Here's how the part is built. I have some questions about the finished solid (model axes, mm). Face numbers are marked on the shaded views. A direction names the side the tool comes from. Coordinates: 2 decimals unless noted, no trailing zeros. Write each loop counter-clockwise with the first axis right and the second up, starting at its lowest first coordinate (ties: lowest second). Pieces come first, ordered by that corner, then holes. Notation, with made-up numbers: M 25.25,88 L 34.25,88 A29 cw 34.25,109 Z; hole C 59.5,47.5 d4. An arc over 180 degrees is marked long. Use a Markdown table: item, result.
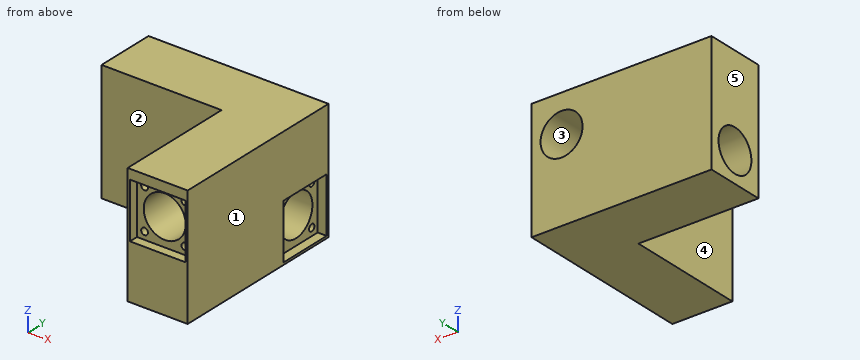
```python
from build123d import *

# Parameters (mm, degrees)
F0_W      = 120
F0_H      = 120
F1_DEPTH  = 80
F2_W      = 37
F2_H      = 37
F2_R      = 2.25
F2_R_2    = 14
F3_DEPTH  = 6
F4_DEPTH  = 120.001
F5_DEPTH  = 25
F6_W      = 37
F6_H      = 37
F6_R      = 2.25
F6_R_2    = 14
F7_DEPTH  = 6
F8_DEPTH  = 120.001
F9_DEPTH  = 25
F10_W     = 80
F10_H     = 80
F11_DEPTH = 80.001


with BuildPart() as f1:
    # F0 (on Top) → F1 (new body)
    with BuildSketch(Plane.XY):
        Rectangle(F0_W, F0_H)
    extrude(amount=F1_DEPTH)

    # F2 (on face) → F3 (cut)
    with BuildSketch(Plane.XZ.offset(60)):
        with Locations((40, 55)):
            Rectangle(F2_W, F2_H)
        with Locations((26.564971, 41.564971)):
            Circle(F2_R, mode=Mode.SUBTRACT)
        with Locations((53.435029, 41.564971)):
            Circle(F2_R, mode=Mode.SUBTRACT)
        with Locations((26.564971, 68.435029)):
            Circle(F2_R, mode=Mode.SUBTRACT)
        with Locations((40, 55)):
            Circle(F2_R_2, mode=Mode.SUBTRACT)
        with Locations((53.435029, 68.435029)):
            Circle(F2_R, mode=Mode.SUBTRACT)
        with Locations((26.564971, 68.435029)):
            Circle(F2_R)
        with Locations((40, 55)):
            Circle(F2_R_2)
        with Locations((53.435029, 68.435029)):
            Circle(F2_R)
        with Locations((53.435029, 41.564971)):
            Circle(F2_R)
        with Locations((26.564971, 41.564971)):
            Circle(F2_R)
    extrude(amount=-F3_DEPTH, mode=Mode.SUBTRACT)

    # F2 (on face) → F4 (cut, through all)
    with BuildSketch(Plane.XZ.offset(60)):
        with Locations((40, 55)):
            Circle(F2_R_2)
    extrude(amount=-F4_DEPTH, mode=Mode.SUBTRACT)

    # F2 (on face) → F5 (cut)
    with BuildSketch(Plane.XZ.offset(60)):
        with Locations((26.564971, 68.435029)):
            Circle(F2_R)
        with Locations((53.435029, 68.435029)):
            Circle(F2_R)
        with Locations((53.435029, 41.564971)):
            Circle(F2_R)
        with Locations((26.564971, 41.564971)):
            Circle(F2_R)
    extrude(amount=-F5_DEPTH, mode=Mode.SUBTRACT)

    # F6 (on face) → F7 (cut)
    with BuildSketch(Plane.YZ.offset(60)):
        with Locations((40, 20)):
            Rectangle(F6_W, F6_H)
        with Locations((26.564971, 6.564971)):
            Circle(F6_R, mode=Mode.SUBTRACT)
        with Locations((53.435029, 6.564971)):
            Circle(F6_R, mode=Mode.SUBTRACT)
        with Locations((26.564971, 33.435029)):
            Circle(F6_R, mode=Mode.SUBTRACT)
        with Locations((40, 20)):
            Circle(F6_R_2, mode=Mode.SUBTRACT)
        with Locations((53.435029, 33.435029)):
            Circle(F6_R, mode=Mode.SUBTRACT)
        with Locations((40, 20)):
            Circle(F6_R_2)
        with Locations((26.564971, 33.435029)):
            Circle(F6_R)
        with Locations((53.435029, 33.435029)):
            Circle(F6_R)
        with Locations((53.435029, 6.564971)):
            Circle(F6_R)
        with Locations((26.564971, 6.564971)):
            Circle(F6_R)
    extrude(amount=-F7_DEPTH, mode=Mode.SUBTRACT)

    # F6 (on face) → F8 (cut, through all)
    with BuildSketch(Plane.YZ.offset(60)):
        with Locations((40, 20)):
            Circle(F6_R_2)
    extrude(amount=-F8_DEPTH, mode=Mode.SUBTRACT)

    # F6 (on face) → F9 (cut)
    with BuildSketch(Plane.YZ.offset(60)):
        with Locations((26.564971, 33.435029)):
            Circle(F6_R)
        with Locations((53.435029, 33.435029)):
            Circle(F6_R)
        with Locations((53.435029, 6.564971)):
            Circle(F6_R)
        with Locations((26.564971, 6.564971)):
            Circle(F6_R)
    extrude(amount=-F9_DEPTH, mode=Mode.SUBTRACT)

    # F10 (on face) → F11 (cut, through all)
    with BuildSketch(Plane.XY.offset(80)):
        with Locations((-20, -20)):
            Rectangle(F10_W, F10_H)
    extrude(amount=-F11_DEPTH, mode=Mode.SUBTRACT)


solid = f1.part
```
1. We'd pull the mould along X, two halves only. Please class the marked faces 1, 2 and 3: +X half, -X half, draft (parallel to the pull), parting line (faces both ways), or undercut.
Answers follow:
| item | result |
|---|---|
| face 1 | +X half |
| face 2 | draft |
| face 3 | undercut |
2. Suppose I cut it at A-A on z = 20. Write out the boundary of the cut face in (x, y).
Answers follow:
| item | result |
|---|---|
| outline | M -60,20 L 20,20 L 20,-60 L 60,-60 L 60,21.5 L 54,21.5 L 54,26 L -60,26 Z; M -60,54 L 54,54 L 54,58.5 L 60,58.5 L 60,60 L -60,60 Z |
3. Suppose I cut it at B-B on y = 40. Write out the boundary of the cut face in (x, z), and give its area (3 significant figures).
Answers follow:
| item | result |
|---|---|
| outline | M -60,0 L 60,0 L 60,1.5 L 54,1.5 L 54,6 L -60,6 Z; M -60,34 L 54,34 L 54,38.5 L 60,38.5 L 60,80 L -60,80 Z; hole C 40,55 d28 |
| area | 5,570 mm2 |
4. Will these pins go through, and if not, where does the flat tip stop? pin 1 Ø25 at (y, z) = (40, 20) entering from -X; pin 2 Ø5 at (y, z) = (25.5, 33.5) entering from +X; pin 3 Ø1.3 at (x, z) = (27, 41) entering from -Y.
Answers follow:
| item | result |
|---|---|
| pin 1 | passes through |
| pin 2 | stops at x = 54 |
| pin 3 | stops at y = -35 |
5. I need wall thicknesses on probe 1 along Z at (x, y) = (-21.5, 40); probe 2 along Y at (x, z) = (-34, 56); probe 3 along Y at (x, z) = (-33, 11). Which ranges of each line are inside material? Lowest first, please.
Answers follow:
| item | result |
|---|---|
| probe 1 | z = 0 to 6, 34 to 80 |
| probe 2 | y = 20 to 60 |
| probe 3 | y = 20 to 29.28, 50.72 to 60 |
6. Suppose I cut it at C-C on x = 40. Write out the boundary of the cut face in (y, z), and give its area (3 significant figures).
Answers follow:
| item | result |
|---|---|
| outline | M -60,0 L 60,0 L 60,41 L -54,41 L -54,36.5 L -60,36.5 Z; M -60,73.5 L -54,73.5 L -54,69 L 60,69 L 60,80 L -60,80 Z; hole C 26.56,6.56 d4.5; hole C 26.56,33.44 d4.5; hole C 40,20 d28; hole C 53.44,6.56 d4.5; hole C 53.44,33.44 d4.5 |
| area | 5,510 mm2 |
7. Suppose I cut it at D-D on x = -22.5. Write out the boundary of the cut face in (y, z), and give its area (3 significant figures).
Answers follow:
| item | result |
|---|---|
| outline | M 20,0 L 60,0 L 60,80 L 20,80 Z; hole C 40,20 d28 |
| area | 2,580 mm2 |
8. Which directions (+Z, -Z, +X, -X, +Y, -Y) give clear straight access to the entire face, cutting with the end or side of a thin tool? Please do the marked faces 4 and 5.
Answers follow:
| item | result |
|---|---|
| face 4 | +Z, -Z, -X, -Y |
| face 5 | +Z, -Z, -X, +Y, -Y |
